Autodesk Inventor part; units mm, degrees
ref_plane "YZ Plane" through (0, 0, 0) normal (1, 0, 0) x (0, 1, 0)
ref_plane "XZ Plane" through (0, 0, 0) normal (0, 1, 0) x (-1, 0, 0)
ref_plane "XY Plane" through (0, 0, 0) normal (0, 0, 1) x (1, 0, 0)
sketch "Sketch1" plane through (0, 0, 0) normal (1, 0, 0) x (0, 1, 0)
  line L0 (-69.85, 342.9) -> (-69.85, -342.9)
  line L1 (-69.85, -342.9) -> (69.85, -342.9)
  line L2 (69.85, -342.9) -> (69.85, 342.9)
  line L3 (69.85, 342.9) -> (-69.85, 342.9)
  line L4 (-69.85, 342.9) -> (69.85, -342.9) construction
  line L5 (-69.85, -342.9) -> (69.85, 342.9) construction
  point P0 (0, 0)
  dimension "width" = 685.8
  dimension "height" = 139.7
extrude "Extrusion1" add sketch "Sketch1" along normal blind 3.175
sketch "Sketch2" plane through (3.175, 0, 0) normal (1, 0, 0) x (0, 0, -1)
  line L0 (-317.5, 38.1) -> (-63.5, 38.1) construction
  line L1 (-317.5, 28.575) -> (-63.5, 28.575)
  line L2 (-63.5, 47.625) -> (-317.5, 47.625)
  arc A0 (-317.5, 47.625) -> (-317.5, 28.575) centre (-317.5, 38.1) ccw
  arc A1 (-63.5, 28.575) -> (-63.5, 47.625) centre (-63.5, 38.1) ccw
  line L3 (342.9, 69.85) -> (-342.9, 69.85)
  line L4 (-342.9, 69.85) -> (-342.9, -69.85)
  line L5 (63.5, -38.1) -> (317.5, -38.1) construction
  line L6 (63.5, -47.625) -> (317.5, -47.625)
  line L7 (317.5, -28.575) -> (63.5, -28.575)
  arc A2 (63.5, -28.575) -> (63.5, -47.625) centre (63.5, -38.1) ccw
  arc A3 (317.5, -47.625) -> (317.5, -28.575) centre (317.5, -38.1) ccw
  line L8 (-342.9, -69.85) -> (342.9, -69.85)
  line L9 (342.9, -69.85) -> (342.9, 69.85)
  point P0 (0, 0)
  point P1 (-190.5, 38.1)
  point P2 (190.5, -38.1)
  dimension "slot_center_from_top" = 31.75
  dimension "slot_center_from_side" = 152.4
  dimension "slot_radius" = 9.525
  dimension "d7" = 31.75
  dimension "d8" = 152.4
  dimension "d9" = 9.525
  dimension "length_of_slot" = 254
  dimension "d13" = 254
extrude "Extrusion2" cut sketch "Sketch2" against normal through all contours A0 L2 A1 L1 | A2 L7 A3 L6
sketch "Sketch3" plane through (0, 0, 0) normal (-1, 0, 0) x (0, 0, 1)
  line L0 (-342.9, 69.85) -> (342.9, 69.85) construction
  line L1 (6.3584, 69.85) -> (6.3584, -72.7678) construction
  line L2 (342.9, 69.85) -> (342.9, -69.85) construction
  line L3 (-6.3584, 69.85) -> (-6.3584, -69.85) construction
  line L4 (-342.9, -69.85) -> (-342.9, 69.85) construction
  line L5 (-6.3584, 61.976) -> (6.3584, 61.976) construction
  line L6 (-6.3584, -61.976) -> (6.3584, -61.976) construction
  line L7 (342.9, -69.85) -> (-342.9, -69.85) construction
  line L8 (-6.3584, 14.224) -> (6.3584, 14.224) construction
  line L9 (-6.3584, -14.224) -> (6.3584, -14.224) construction
  point P0 (0, 0)
  point P1 (80.6051, 237.827)
  point P2 (47.886, -92.9067)
  dimension "Vertical_Line_For_Bolt_Holes" = 336.5416
  dimension "d15" = 336.5416
  dimension "First_Horizontal_Line" = 7.874
  dimension "d17" = 7.874
  dimension "Second_Horizontal_Line" = 47.752
  dimension "d19" = 47.752
hole "Hole1" at (0, 61.976, 6.3584) at (0, -61.976, -6.3584) at (0, 237.827, 80.6051) at (0, -92.9067, 47.886) at (0, 14.224, 6.3584) at (0, -14.224, -6.3584) direction (1, 0, 0) diameter 6.35 end through all
equation "\"d9\" = slot_radius"
equation "\"d13\" = length_of_slot"
equation "\"d15\" = Vertical_Line_For_Bolt_Holes"
equation "\"d17\" = First_Horizontal_Line"
properties part number "5.5 x 27 x 1/8 x 3/8" material "Polyethylene, High Density"
Build history of the part. All positions in model axes, mm. Coordinates: 2 decimals unless noted, no trailing zeros. Order: outer loops, then holes, each group sorted by start corner. A loop starts at its lowest first (then second) coordinate and runs counter-clockwise, first axis right, second up. Notation, with made-up numbers: (-11, -37.5) -> (21, -37.5) arc R29 ccw to (21, -13.5) -> close; hole circle Ø1 at (8.5, 22.25). An arc over 180 degrees is marked (long way). Answer in a Markdown table with one row per item. Add a question column.
Q1. Drop flat-ended pins along their axis: pin 1 (8 mm diameter, centred on y = 14.5, z = -46.5, fed in from -X); pin 2 (5 mm diameter, centred on y = -14.22, z = -6.36, fed in from +X). Give the stop position or say it passes through.
Q2. Band-saw the part on C-C, the plane x = 2.6. List the corners of the cut face in (y, z) (3 decimals).
Q3. Band-saw the part on B-B, the plane z = -200.5. List the corners of the cut face in (x, y) (3 decimals).
Q4. Band-saw the part on A-A, the plane y = 38.1. List the corners of the cut face in (x, z) (3 decimals).
Q5. Wall check: line 1 along Y through (x, z) = (2.6, -169) (3 decimals); line 2 along Y through (x, z) = (2.5, 313.5) (3 decimals); line 3 along Y through (x, z) = (0.65, 4). Give the ranges that are in metal, low to high. Write a range as [from, to].
Answers follow:
| question | item | result |
|---|---|---|
| 1 | pin 1 | x = 0 |
| 1 | pin 2 | through |
| 2 | outline | (-69.85, -342.9) -> (69.85, -342.9) -> (69.85, 342.9) -> (-69.85, 342.9) -> close; hole circle Ø6.35 at (-61.976, -6.358); hole (-47.625, -317.5) arc R9.525 ccw to (-28.575, -317.5) -> (-28.575, -63.5) arc R9.525 ccw to (-47.625, -63.5) -> close; hole circle Ø6.35 at (-14.224, -6.358); hole circle Ø6.35 at (14.224, 6.358); hole (28.575, 63.5) arc R9.525 ccw to (47.625, 63.5) -> (47.625, 317.5) arc R9.525 ccw to (28.575, 317.5) -> close; hole circle Ø6.35 at (61.976, 6.358) |
| 3 | outline | (0, -69.85) -> (3.175, -69.85) -> (3.175, -47.625) -> (0, -47.625) -> close; (0, -28.575) -> (3.175, -28.575) -> (3.175, 69.85) -> (0, 69.85) -> close |
| 4 | outline | (0, -342.9) -> (3.175, -342.9) -> (3.175, 53.975) -> (0, 53.975) -> close; (0, 327.025) -> (3.175, 327.025) -> (3.175, 342.9) -> (0, 342.9) -> close |
| 5 | line 1 | [-69.85, -47.625], [-28.575, 69.85] |
| 5 | line 2 | [-69.85, 28.575], [47.625, 69.85] |
| 5 | line 3 | [-69.85, 12.1], [16.35, 59.85], [64.1, 69.85] |
